Check sheet for the drawn part. Datum: minimum x, y, z corner. Units: mm. Coordinates: 2 decimals unless noted, no trailing zeros. Write each loop counter-clockwise with the first axis right and the second up, starting at its lowest first coordinate (ties: lowest second). Pieces come first, ordered by that corner, then holes. Notation, with made-up numbers: (-38.5, 67) -> (1.5, 67) arc R26 ccw to (1.5, 94) -> close; hole circle Ø6 at (-6, 69.5). An arc over 180 degrees is marked (long way). One line per question, with ' | ' between items.
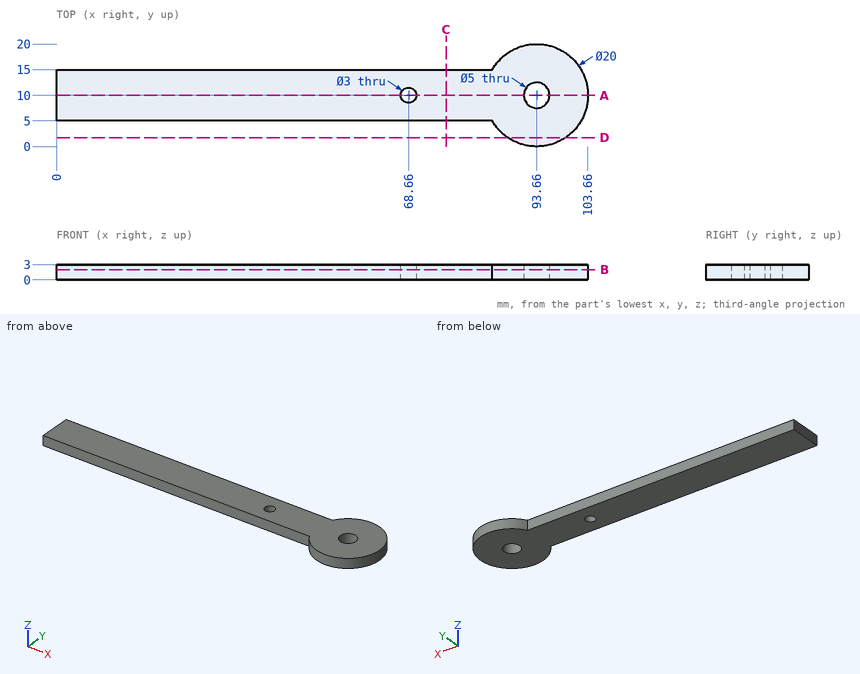
1. Material ranges on line 1 (X direction, y = 9.5, z = 1.1) (1 decimal); line 2 (Y direction, x = 13.5, z = 2.3); line 3 (Y direction, x = 87, z = 2.6), recorded low to high. Write a range as from..to.
Worked answers:
line 1: 0..67.2, 70.1..91.2, 96.1..103.6 | line 2: 5..15 | line 3: 2.54..17.46
2. Go/stop test with flat-tipped pins: P1, Ø6, axis at x = 25.5, y = 8, coming from the -Z side; P2, Ø0.9, axis at x = 27, z = 2, coming from the -Y side; P3, Ø1, axis at x = 66.5, z = 2, coming from the +Y side. Record where each tip stops, or that it passes through.
Worked answers:
P1: z = 0 | P2: y = 5 | P3: y = 15
3. Cross-section at B-B on z = 2. Record the boundary of the cut face in (x, y), and give its area (3 significant figures).
Worked answers:
outline: (0, 5) -> (85, 5) arc R10 ccw (long way) to (85, 15) -> (0, 15) -> close; hole circle Ø3 at (68.66, 10); hole circle Ø5 at (93.66, 10) | area: 1,130 mm²
4. Cross-section at D-D on y = 1.75. Record the boundary of the cut face in (x, z).
Worked answers:
outline: (88.01, 0) -> (99.31, 0) -> (99.31, 3) -> (88.01, 3) -> close
5. Cross-section at C-C on x = 76. Record the boundary of the cut face in (y, z).
Worked answers:
outline: (5, 0) -> (15, 0) -> (15, 3) -> (5, 3) -> close
6. Cross-section at A-A on y = 10. Record the boundary of the cut face in (x, z).
Worked answers:
outline: (0, 0) -> (67.16, 0) -> (67.16, 3) -> (0, 3) -> close; (70.16, 0) -> (91.16, 0) -> (91.16, 3) -> (70.16, 3) -> close; (96.16, 0) -> (103.66, 0) -> (103.66, 3) -> (96.16, 3) -> close
